Read the model definition and answer for the solid it produces. Units are mm, in the model's axes. A direction names the side the tool comes from. Give positions to 0.01 mm unless a question says otherwise; leave off trailing zeros. Order: outer loops, then holes, each group sorted by start corner. A loop starts at its lowest first (then second) coordinate and runs counter-clockwise, first axis right, second up. Notation, with made-up numbers: (84, 12) - (140, 12) arc R9 cw to (140, 29) - close; hole circle Ø7 at (-30, 43.5). An arc over 180 degrees is marked (long way). Write item = value, one per line.
Autodesk Inventor part; units mm, degrees
ref_plane "YZ Plane" through (0, 0, 0) normal (1, 0, 0) x (0, 1, 0)
ref_plane "XZ Plane" through (0, 0, 0) normal (0, 1, 0) x (-1, 0, 0)
ref_plane "XY Plane" through (0, 0, 0) normal (0, 0, 1) x (1, 0, 0)
sketch "Sketch1" plane through (0, 0, 0) normal (0, 1, 0) x (-1, 0, 0)
  line L0 (0, 0) -> (-60, 0)
  line L1 (-60, 0) -> (-60, -6)
  line L2 (-60, -6) -> (0, -6)
  line L3 (0, -6) -> (0, 0)
  line L4 (-60, 0) -> (-54, 0)
  line L5 (-54, 0) -> (-54, -85)
  line L6 (-54, -85) -> (-60, -85)
  line L7 (-60, -85) -> (-60, 0)
  line L8 (-54, -85) -> (-84, -85)
  line L9 (-84, -85) -> (-84, -79)
  line L10 (-84, -79) -> (-54, -79)
  line L11 (-54, -79) -> (-54, -85)
  point P0 (-60, -79)
  point P1 (-54, -6)
  dimension "d2" = 60
  dimension "d3" = 6
  dimension "d4" = 6
  dimension "d5" = 85
  dimension "d6" = 30
  dimension "d7" = 6
extrude "Extrusion1" add sketch "Sketch1" along normal blind 20
fillet "Fillet1" radius 5 4 edges at (54, 10, -6) (60, 10, 0) (60, 10, -79) (54, 10, -85)
fillet "Fillet2" radius 1.5 4 edges at (0, 10, -6) (0, 10, 0) (84, 10, -85) (84, 10, -79)
sketch "Sketch2" plane through (49, 0, -6) normal (0, 0, -1) x (-1, 0, 0)
  line L0 (47.5, 0) -> (47.5, 20)
  line L1 (47.5, 10) -> (22.5, 10)
  line L2 (0, 0) -> (0, 20)
  line L3 (7.5, 10) -> (37.5, 10) construction
  line L4 (7.5, 7) -> (37.5, 7)
  line L5 (37.5, 13) -> (7.5, 13)
  arc A0 (7.5, 13) -> (7.5, 7) centre (7.5, 10) ccw
  arc A1 (37.5, 7) -> (37.5, 13) centre (37.5, 10) ccw
  point P0 (49, 0)
  dimension "d12" = 25
  dimension "d13" = 15
  dimension "d14" = 6
extrude "Extrusion2" cut sketch "Sketch2" against normal through all
sketch "Sketch3" plane through (59, 0, -85) normal (0, 0, -1) x (-1, 0, 0)
  line L0 (-23.5, 0) -> (-23.5, 20)
  line L1 (-23.5, 10) -> (-13.5, 10)
  line L2 (0, 20) -> (0, 0)
  circle A0 centre (-13.5, 10) radius 3
  point P0 (59, 0)
  dimension "d17" = 10
  dimension "d18" = 6
extrude "Extrusion3" cut sketch "Sketch3" against normal through all
properties part number "PowerBrick_Clamp"
1. Section D-D (z = -50.5) is taken. Determine the outline of the cut face in (x, y).
Recorded:
outline = (54, 0) - (60, 0) - (60, 20) - (54, 20) - close
2. Section B-B (y = 10) is taken. Determine the outline of the cut face in (x, z), and give its area (3 significant figures).
Recorded:
outline = (0, -4.5) arc R1.5 ccw to (1.5, -6) - (8.5, -6) - (8.5, 0) - (1.5, 0) arc R1.5 ccw to (0, -1.5) - close; (44.5, -6) - (49, -6) arc R5 cw to (54, -11) - (54, -80) arc R5 ccw to (59, -85) - (69.5, -85) - (69.5, -79) - (65, -79) arc R5 cw to (60, -74) - (60, -5) arc R5 ccw to (55, 0) - (44.5, 0) - close; (75.5, -85) - (82.5, -85) arc R1.5 ccw to (84, -83.5) - (84, -80.5) arc R1.5 ccw to (82.5, -79) - (75.5, -79) - close
area = 724 mm^2
3. Determine the mould class of faces 6 (the face through (55, 0, -33)), 7 (the face through (0, 10, -3)), 8 (the face through (55, 20, -33)), 9 (the face through (27, 7, -3)) for opening direction Y: +Y half, -Y half, draft (parallel to the pull), parting line (faces both ways), or undercut.
Recorded:
face_6 = -Y half
face_7 = draft
face_8 = +Y half
face_9 = undercut
4. Flat-ended cylindrical pins translate along their axes: pin 1 (8 mm diameter, centred on x = 72.5, y = 10, fed in from +Z); pin 2 (1.5 mm diameter, centred on x = 60, y = 14, fed in from +Z); pin 3 (6 mm diameter, centred on x = 43, y = 16.5, fed in from -Z). Find the tip coordinate at first contact, or state that the pin passes through.
Recorded:
pin_1 = -79
pin_2 = -2.37
pin_3 = -6
5. Section A-A (x = 72.5) is taken. Determine the outline of the cut face in (y, z).
Recorded:
outline = (0, -85) - (7, -85) - (7, -79) - (0, -79) - close; (13, -85) - (20, -85) - (20, -79) - (13, -79) - close
6. Section C-C (y = 2.5) is taken. Determine the outline of the cut face in (x, z).
Recorded:
outline = (0, -4.5) arc R1.5 ccw to (1.5, -6) - (49, -6) arc R5 cw to (54, -11) - (54, -80) arc R5 ccw to (59, -85) - (82.5, -85) arc R1.5 ccw to (84, -83.5) - (84, -80.5) arc R1.5 ccw to (82.5, -79) - (65, -79) arc R5 cw to (60, -74) - (60, -5) arc R5 ccw to (55, 0) - (1.5, 0) arc R1.5 ccw to (0, -1.5) - close
7. For faces 1 (the face through (44.5, 10.1, -3)), 2 (the face through (84, 10, -82)), 3 (the face through (76, 10, -79)), 4 (the face through (28, 5, 0)), 5 (the face through (26, 5, -6)), determine the directions among +Z, -Z, +X, -X, +Y, -Y from which every point of the face is accessible in a straight line to the end or side of a thin tool.
Recorded:
face_1 = +Z, -Z
face_2 = +Z, -Z, +X, +Y, -Y
face_3 = +Z, +X, +Y, -Y
face_4 = +Z, +X, -X, +Y, -Y
face_5 = -Z, -X, +Y, -Y
8. Straight lines are drawn through the part: L1, parallel to Y at x = 72.5, z = -83.55; L2, parallel to X at y = 10, z = -80.4; L3, parallel to Z at x = 31.5, y = 6. For each, find the intervals that lie inside material, in ascending order. Write a range as [from, to].
Recorded:
L1 = [0, 7], [13, 20]
L2 = [54.02, 69.5], [75.5, 84]
L3 = [-6, 0]
